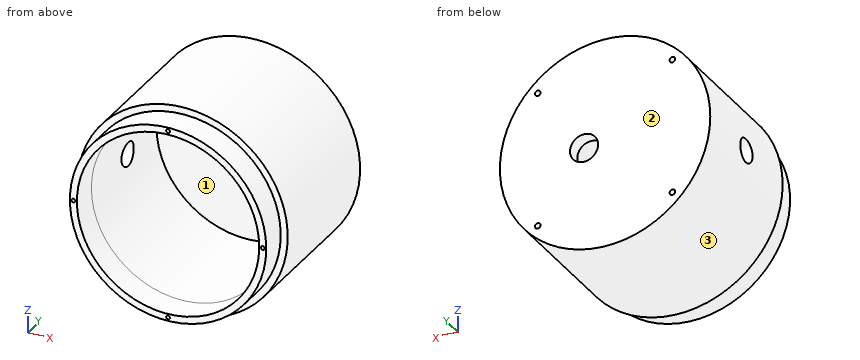
Autodesk Inventor part; units mm, degrees
ref_plane "작업 평면1" through (0, -20, 0) normal (0, 1, 0) x (-1, 0, 0)
ref_plane "YZ Plane" through (0, 0, 0) normal (1, 0, 0) x (0, 1, 0)
ref_plane "XY Plane" through (0, 0, 0) normal (0, 0, 1) x (1, 0, 0)
sketch "스케치2" plane through (0, 0, 0) normal (0, 1, 0) x (-1, 0, 0)
  circle A0 centre (0, 0) radius 75
  dimension "d1" = 150
extrude "돌출1" add sketch "스케치2" along normal blind 100
shell "쉘1" thickness 10 removed faces 1 at (-17.7208, 0, 28.0232)
sketch "스케치4" plane through (0, 0, 0) normal (0, -1, 0) x (1, 0, 0)
  circle A0 centre (0, 0) radius 65
  circle A1 centre (0, 0) radius 70
  dimension "d10" = 140
extrude "돌출3" add sketch "스케치4" along normal blind 20
ref_plane "작업 평면1" through (0, -20, 0) normal (0, 1, 0) x (-1, 0, 0)
sketch "스케치5" plane through (0, -20, 0) normal (0, 1, 0) x (-1, 0, 0)
  circle A0 centre (-67.5, 0) radius 1.35
  circle A1 centre (0, -67.5) radius 1.35
  circle A2 centre (67.5, 0) radius 1.35
  circle A3 centre (0, 67.5) radius 1.35
  point P0 (0, 0)
  point P1 (0, -67.5)
  point P2 (0, 0)
  point P3 (67.5, 0)
  point P4 (0, 0)
  point P5 (0, 67.5)
  point P6 (0, 0)
  point P7 (0, 0)
  dimension "d17" = 360
  dimension "d71" = 360
sketch "스케치7" plane through (0, 100, 0) normal (0, 1, 0) x (1, 0, 0)
  circle A0 centre (15, 0) radius 10
  point P0 (0, 0)
  dimension "d45" = 20
  dimension "d46" = 15
extrude "돌출4" cut sketch "스케치7" against normal blind 10
sketch "스케치8" plane through (0, 0, 0) normal (1, 0, 0) x (0, 1, 0)
  circle A0 centre (50, 0) radius 8.5
  line L0 (0, 75) -> (0, -75)
  point P0 (0, 0)
  dimension "d30" = 17
  dimension "d31" = 50
extrude "돌출5" cut sketch "스케치8" against normal through all
sketch "스케치12" plane through (0, 100, 0) normal (0, 1, 0) x (1, 0, 0)
  circle A0 centre (15, 0) radius 10
  circle A1 centre (48, -48) radius 2
  circle A2 centre (-48, -48) radius 2
  circle A3 centre (48, 48) radius 2
  circle A4 centre (-48, 48) radius 2
  line L0 (48, 48) -> (-48, -48) construction
  line L1 (-48, 48) -> (48, -48) construction
  point P0 (0, 0)
  dimension "d66" = 4
  dimension "d75" = 96
  dimension "d76" = 96
extrude "돌출8" cut sketch "스케치12" against normal blind 10 contours A1 | A2 | A3 | A4
extrude "돌출9" cut sketch "스케치5" along normal blind 8
properties part number "바텀(상)"
Build history of the part. All positions in model axes, mm. Face numbers are marked on the shaded views. Round coordinates to 2 decimals unless told otherwise and drop trailing zeros. Write each loop counter-clockwise with the first axis right and the second up, starting at its lowest first coordinate (ties: lowest second). Pieces come first, ordered by that corner, then holes. Notation, with made-up numbers: (-33.75, 21) -> (22.25, 21) arc R25 cw to (22.25, 53) -> close; hole circle Ø5 at (8, -22.75). An arc over 180 degrees is marked (long way). Use one line per item in the form item = value.
Q1. Band-saw the part on B-B, the plane y = 19.5. Write the cut outline in (x, z).
Conclusion:
outline = circle Ø150 at (0, 0); hole circle Ø130 at (0, 0)
Q2. Band-saw the part on D-D, the plane z = -26. Write the cut outline in (x, y).
Conclusion:
outline = (-70.35, 0) -> (-64.99, 0) -> (-64.99, -20) -> (-59.57, -20) -> (-59.57, 90) -> (59.57, 90) -> (59.57, -20) -> (64.99, -20) -> (64.99, 0) -> (70.35, 0) -> (70.35, 100) -> (-70.35, 100) -> close
Q3. Drop flat-ended pins along their axis: P1, Ø1.5, axis at x = 3.5, y = 27, coming from the -Z side; P2, Ø3, axis at x = -43, y = 6.5, coming from the -Z side; P3, Ø5, axis at y = 87, z = -50.5, coming from the +X side. Give the stop position or say it passes through.
Conclusion:
P1 = -74.95
P2 = -62.47
P3 = 57.63
Q4. Band-saw the part on C-C, the plane x = 48. Write the cut outline in (y, z), then the cut area to 3 significant figures.
Conclusion:
outline = (-20, -50.95) -> (0, -50.95) -> (0, -57.63) -> (100, -57.63) -> (100, -50) -> (90, -50) -> (90, -46) -> (100, -46) -> (100, 46) -> (90, 46) -> (90, 50) -> (100, 50) -> (100, 57.63) -> (0, 57.63) -> (0, 50.95) -> (-20, 50.95) -> (-20, 43.83) -> (90, 43.83) -> (90, -43.83) -> (-20, -43.83) -> close
area = 3,840 mm²
Q5. Drill centre lines: L1, parallel to Z at x = -49, y = 95.5; L2, parallel to Y at x = 38, z = 32.5; L3, parallel to Z at x = -48, y = 95.75. Where is each one in solid material? Low to high.
Conclusion:
L1 = -56.78 to -49.73, -46.27 to 46.27, 49.73 to 56.78
L2 = 90 to 100
L3 = -57.63 to -50, -46 to 46, 50 to 57.63
Q6. Two-plate mould, pull along Z, no slides. Class the marked faces 1, 2 and 3: released by +Z, released by -Z, zero draft, split by the parting line, or undercut.
Conclusion:
face_1 = undercut
face_2 = zero draft
face_3 = split by the parting line
Q7. Band-saw the part on A-A, the plane x = 15. Write the cut outline in (y, z).
Conclusion:
outline = (-20, -68.37) -> (0, -68.37) -> (0, -73.48) -> (100, -73.48) -> (100, -10) -> (90, -10) -> (90, -63.25) -> (-20, -63.25) -> close; (-20, 63.25) -> (90, 63.25) -> (90, 10) -> (100, 10) -> (100, 73.48) -> (0, 73.48) -> (0, 68.37) -> (-20, 68.37) -> close
